Here's how the part is built. I have some questions about the finished solid (model axes, mm). Face numbers are marked on the shaded views. Round coordinates to 2 decimals unless told otherwise and drop trailing zeros. Loops run counter-clockwise (first coordinate to the right, second up) from the corner with the lowest first, then second, coordinate; pieces in that order, holes last. Notation, with made-up numbers: M -31,83 L 6,83 A28 cw 6,118 Z; hole C 7.25,75 d4. An arc over 180 degrees is marked long. Answer as a JSON object with one key per item and string values.
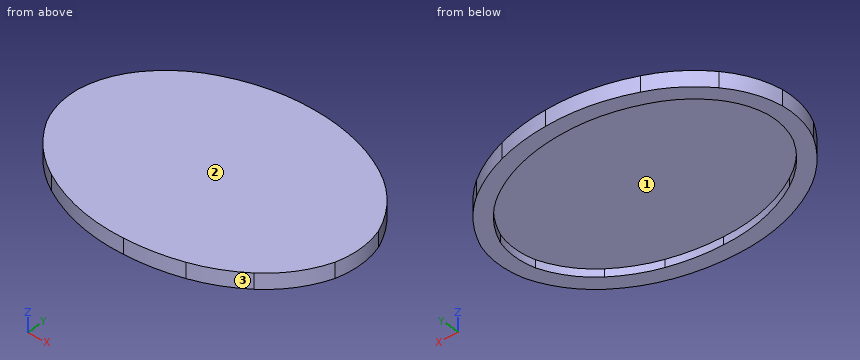
from build123d import *

# Parameters (mm, degrees)
BOSS_EXTRUDE1_DEPTH = 1
BOSS_EXTRUDE2_START = -2
BOSS_EXTRUDE2_DEPTH = 2
BOSS_EXTRUDE3_START = 2
BOSS_EXTRUDE3_DEPTH = 2


with BuildPart() as part:
    # Sketch2 → Boss-Extrude1 (new body)
    with BuildSketch(Plane.XY):
        with BuildLine():
            ThreePointArc((14.582306461, -23.937478676), (20.662688223, -21.536481735), (26.227582561, -18.10606198))
            ThreePointArc((26.227582561, -18.10606198), (31.602803157, -12.702637223), (35.175830441, -5.970366314))
            ThreePointArc((35.175830441, -5.970366314), (35.940455788, 0.032211939), (34.924872534, 5.997460321))
            ThreePointArc((34.924872534, 5.997460321), (30.999615253, 12.739070672), (25.401678251, 18.172306925))
            ThreePointArc((25.401678251, 18.172306925), (20.023450582, 21.36826462), (14.22923276, 23.727611624))
            ThreePointArc((14.22923276, 23.727611624), (7.882073391, 25.295796991), (1.378547715, 25.966461733))
            ThreePointArc((1.378547715, 25.966461733), (-9.069964823, 25.28846457), (-19.084442092, 22.232104078))
            ThreePointArc((-19.084442092, 22.232104078), (-25.480773521, 18.669901445), (-30.847619904, 13.690011561))
            ThreePointArc((-30.847619904, 13.690011561), (-34.216625408, 8.281245191), (-35.888880176, 2.132382229))
            ThreePointArc((-35.888880176, 2.132382229), (-35.572811659, -3.288450427), (-33.85309471, -8.438974634))
            ThreePointArc((-33.85309471, -8.438974634), (-28.98576201, -14.979441817), (-22.570123581, -20.01016961))
            ThreePointArc((-22.570123581, -20.01016961), (-11.367274893, -24.644691823), (0.679303276, -26.009451613))
            ThreePointArc((0.679303276, -26.009451613), (7.703427235, -25.460763497), (14.582306461, -23.937478676))
        make_face()
    extrude(amount=BOSS_EXTRUDE1_DEPTH)

    # Sketch3 → Boss-Extrude2 (add)
    with BuildSketch(Plane.XY.offset(1).offset(BOSS_EXTRUDE2_START)):
        with BuildLine():
            ThreePointArc((-23.584596954, -21.733783191), (-11.876170523, -26.578887071), (0.714158664, -28.009233893))
            ThreePointArc((0.714158664, -28.009233893), (8.007585987, -27.437521821), (15.150208477, -25.855156256))
            ThreePointArc((15.150208477, -25.855156256), (21.558193731, -23.324796552), (27.422917732, -19.709549999))
            ThreePointArc((27.422917732, -19.709549999), (33.232049111, -13.863052711), (37.082922231, -6.576193708))
            ThreePointArc((37.082922231, -6.576193708), (37.93992708, 0.078373421), (36.802232938, 6.690738583))
            ThreePointArc((36.802232938, 6.690738583), (32.590590722, 13.951259274), (26.567668782, 19.797412042))
            ThreePointArc((26.567668782, 19.797412042), (20.924163176, 23.153997512), (14.843057348, 25.631087228))
            ThreePointArc((14.843057348, 25.631087228), (8.234147075, 27.264583601), (1.462460857, 27.964777266))
            ThreePointArc((1.462460857, 27.964777266), (-9.426205562, 27.256483976), (-19.863550161, 24.074256219))
            ThreePointArc((-19.863550161, 24.074256219), (-26.665599434, 20.281211791), (-32.373640199, 14.982784573))
            ThreePointArc((-32.373640199, 14.982784573), (-36.059000484, 9.059793769), (-37.879998788, 2.325726228))
            ThreePointArc((-37.879998788, 2.325726228), (-37.536082018, -3.670000019), (-35.627002731, -9.364069587))
            ThreePointArc((-35.627002731, -9.364069587), (-30.435882217, -16.357044434), (-23.584596954, -21.733783191))
        make_face()
        with BuildLine():
            ThreePointArc((-22.570123581, -20.01016961), (-11.367274893, -24.644691823), (0.679303276, -26.009451613))
            ThreePointArc((0.679303276, -26.009451613), (7.703427235, -25.460763497), (14.582306461, -23.937478676))
            ThreePointArc((14.582306461, -23.937478676), (20.662688223, -21.536481735), (26.227582561, -18.10606198))
            ThreePointArc((26.227582561, -18.10606198), (31.602803157, -12.702637223), (35.175830441, -5.970366314))
            ThreePointArc((35.175830441, -5.970366314), (35.940455788, 0.032211939), (34.924872534, 5.997460321))
            ThreePointArc((34.924872534, 5.997460321), (30.999615253, 12.739070672), (25.401678251, 18.172306925))
            ThreePointArc((25.401678251, 18.172306925), (20.023450582, 21.36826462), (14.22923276, 23.727611624))
            ThreePointArc((14.22923276, 23.727611624), (7.882073391, 25.295796991), (1.378547715, 25.966461733))
            ThreePointArc((1.378547715, 25.966461733), (-9.069964823, 25.28846457), (-19.084442092, 22.232104078))
            ThreePointArc((-19.084442092, 22.232104078), (-25.480773521, 18.669901445), (-30.847619904, 13.690011561))
            ThreePointArc((-30.847619904, 13.690011561), (-34.216625408, 8.281245191), (-35.888880176, 2.132382229))
            ThreePointArc((-35.888880176, 2.132382229), (-35.572811659, -3.288450427), (-33.85309471, -8.438974634))
            ThreePointArc((-33.85309471, -8.438974634), (-28.98576201, -14.979441817), (-22.570123581, -20.01016961))
        make_face(mode=Mode.SUBTRACT)
    extrude(amount=BOSS_EXTRUDE2_DEPTH)

    # Sketch4 → Boss-Extrude3 (add)
    with BuildSketch(Plane(origin=(0, 0, -1), x_dir=(-1, 0, 0), z_dir=(0, 0, -1)).offset(BOSS_EXTRUDE3_START)):
        with BuildLine():
            ThreePointArc((23.584596954, -21.733783191), (30.435882217, -16.357044434), (35.627002731, -9.364069587))
            ThreePointArc((35.627002731, -9.364069587), (37.536082018, -3.670000019), (37.879998788, 2.325726228))
            ThreePointArc((37.879998788, 2.325726228), (36.059000484, 9.059793769), (32.373640199, 14.982784573))
            ThreePointArc((32.373640199, 14.982784573), (26.665599434, 20.281211791), (19.863550161, 24.074256219))
            ThreePointArc((19.863550161, 24.074256219), (9.426205562, 27.256483976), (-1.462460857, 27.964777266))
            ThreePointArc((-1.462460857, 27.964777266), (-8.234147075, 27.264583601), (-14.843057348, 25.631087228))
            ThreePointArc((-14.843057348, 25.631087228), (-20.924163176, 23.153997512), (-26.567668782, 19.797412042))
            ThreePointArc((-26.567668782, 19.797412042), (-32.590590722, 13.951259274), (-36.802232938, 6.690738583))
            ThreePointArc((-36.802232938, 6.690738583), (-37.93992708, 0.078373421), (-37.082922231, -6.576193708))
            ThreePointArc((-37.082922231, -6.576193708), (-33.232049111, -13.863052711), (-27.422917732, -19.709549999))
            ThreePointArc((-27.422917732, -19.709549999), (-21.558193731, -23.324796552), (-15.150208477, -25.855156256))
            ThreePointArc((-15.150208477, -25.855156256), (-8.007585987, -27.437521821), (-0.714158664, -28.009233893))
            ThreePointArc((-0.714158664, -28.009233893), (11.876170523, -26.578887071), (23.584596954, -21.733783191))
        make_face()
        with BuildLine():
            ThreePointArc((21.555650209, -18.286556029), (27.535330411, -13.602126211), (32.078697256, -7.514575328))
            ThreePointArc((32.078697256, -7.514575328), (33.609473864, -2.907248333), (33.897648559, 1.939162133))
            ThreePointArc((33.897648559, 1.939162133), (32.374200723, 7.502749449), (29.321599609, 12.39723855))
            ThreePointArc((29.321599609, 12.39723855), (24.296047221, 17.05851306), (18.305561132, 20.389839116))
            ThreePointArc((18.305561132, 20.389839116), (8.713855119, 23.320421058), (-1.294621046, 23.968139818))
            ThreePointArc((-1.294621046, 23.968139818), (-7.529992858, 23.327009842), (-13.615408172, 21.82413602))
            ThreePointArc((-13.615408172, 21.82413602), (-19.122622483, 19.582585616), (-24.235471698, 16.547337587))
            ThreePointArc((-24.235471698, 16.547337587), (-29.408223084, 11.527376998), (-33.046936389, 5.305068206))
            ThreePointArc((-33.046936389, 5.305068206), (-33.940979932, -0.013771926), (-33.268351754, -5.365121806))
            ThreePointArc((-33.268351754, -5.365121806), (-29.973321616, -11.542469618), (-25.032247389, -16.502573961))
            ThreePointArc((-25.032247389, -16.502573961), (-19.767182716, -19.748166918), (-14.014404446, -22.019801096))
            ThreePointArc((-14.014404446, -22.019801096), (-7.399238865, -23.484007784), (-0.644388471, -24.00966267))
            ThreePointArc((-0.644388471, -24.00966267), (10.858407416, -22.710487179), (21.555650209, -18.286556029))
        make_face(mode=Mode.SUBTRACT)
    extrude(amount=-BOSS_EXTRUDE3_DEPTH)


solid = part.part
Item 1: Please list where these lines run through material, in increasing order: probe 1 along Z at (x, y) = (17, -10); probe 2 along X at (y, z) = (-9.5, -0.1); probe 3 along X at (y, z) = (-18.5, -1.85). Write a range as from..to.
Resolved:
{"probe 1": "0..1", "probe 2": "-35.55..-33.24, 33.62..35.86", "probe 3": "-28.14..-21.19, 22.05..28.93"}
Item 2: I want a section at B-B, the plane x = -17. Please give me the cut outline in (y, z).
Resolved:
{"outline": "M -24.93,-3 L -20.6,-3 L -20.6,-1 L -22.77,-1 L -22.77,0 L 23.08,0 L 23.08,-1 L 20.94,-1 L 20.94,-3 L 25.21,-3 L 25.21,1 L -24.93,1 Z"}
Item 3: If we mould it in two halves opening along Y, with no side actions, what happens to the marked faces 1, 2 and 3? For each: pulls with the +Y half, pulls with the -Y half, needs draft (parallel to the pull), parting line crosses it, or undercut.
Resolved:
{"face 1": "undercut", "face 2": "needs draft", "face 3": "pulls with the -Y half"}
Item 4: I want a section at A-A, the plane z = -1.7. Please give me the cut outline in (x, y), then the cut area to 3 significant figures.
Resolved:
{"outline": "M -37.88,2.33 A22.63 ccw -35.63,-9.36 A32.74 ccw -23.58,-21.73 A45.53 ccw 0.71,-28.01 A52.38 ccw 15.15,-25.86 A39.12 ccw 27.42,-19.71 A27.94 ccw 37.08,-6.58 A22.56 ccw 36.8,6.69 A30.66 ccw 26.57,19.8 A43.89 ccw 14.84,25.63 A48.92 ccw 1.46,27.96 A47.35 ccw -19.86,24.07 A32.59 ccw -32.37,14.98 A23.94 ccw Z; hole M -33.9,1.94 A18.63 ccw -32.08,-7.51 A28.74 ccw -21.56,-18.29 A41.53 ccw 0.64,-24.01 A48.38 ccw 14.01,-22.02 A35.12 ccw 25.03,-16.5 A23.94 ccw 33.27,-5.37 A18.56 ccw 33.05,5.31 A26.66 ccw 24.24,16.55 A39.89 ccw 13.62,21.82 A44.92 ccw 1.29,23.97 A43.35 ccw -18.31,20.39 A28.59 ccw -29.32,12.4 A19.94 ccw Z", "area": "784 mm²"}
Item 5: I want a section at C-C, the plane y = 11.5. Please give me the cut outline in (x, z), then the cut area to 3 significant figures.
Resolved:
{"outline": "M -34.83,-3 L -30.04,-3 L -30.04,-1 L -32.48,-1 L -32.48,0 L 31.92,0 L 31.92,-1 L 29.43,-1 L 29.43,-3 L 34.32,-3 L 34.32,1 L -34.83,1 Z", "area": "93.3 mm²"}
Item 6: I'm going to push a flat-ended pin straight in: pin 1 Ø5 at (x, y) = (12, 11.5) entering from -Z. Where does the tip first touch, or does it pass through?
Resolved:
{"pin 1": "z = 0"}
